Work out the finished part from the listing and answer in its coordinate system (mm). Face numbers are marked on the shaded views. A direction names the side the tool comes from. Coordinates: 2 decimals unless noted, no trailing zeros. Order: outer loops, then holes, each group sorted by start corner. A loop starts at its lowest first (then second) coordinate and runs counter-clockwise, first axis right, second up. Notation, with made-up numbers: M 83,73 L 132,73 A21 ccw 132,84 Z; hole C -5,34.25 d9. An arc over 180 degrees is marked long. Write item = value, one per line. Start each with the question number.
Q1. Determine the mould class of the marked faces 6, 7 and 8 for opening direction X: released by +X, released by -X, zero draft, split by the parting line, or undercut.
Q2. A tool of negligible diameter and unlimited length cuts with its end or side. For the marked faces 1, 2, 3, 4 and 5, from which of +Z, -Z, +X, -X, +Y, -Y can it reach the whole face along a straight path? Write none if from no direction.
Q3. Find section C-C on y = 51. Give the vertices of the cut face in (x, z).
Q4. Find section D-D on y = 101. Give the vertices of the cut face in (x, z), and give its area (3 significant figures).
Q5. Each of these flat-tipped pins is pushed along its axis until it touches: P1, Ø10, axis at y = 42, z = -19, coming from the -X side; P2, Ø3, axis at y = 87, z = -14.5, coming from the +X side; P3, Ø14.5, axis at y = 11.5, z = -42.5, coming from the +X side. Where does it stop, or does it pass through?
Q6. Find section B-B on x = -40. Give the vertices of the cut face in (y, z).
Q7. Straight lines are drawn through the part: line 1 along X through (y, z) = (6.5, -72); line 2 along Z through (x, y) = (57, 103); line 3 along Y through (x, z) = (84, -51). For each, find the intervals that lie inside material, in ascending order.
Q8. Find section A-A on z = -46. Give the vertices of the cut face in (x, y).
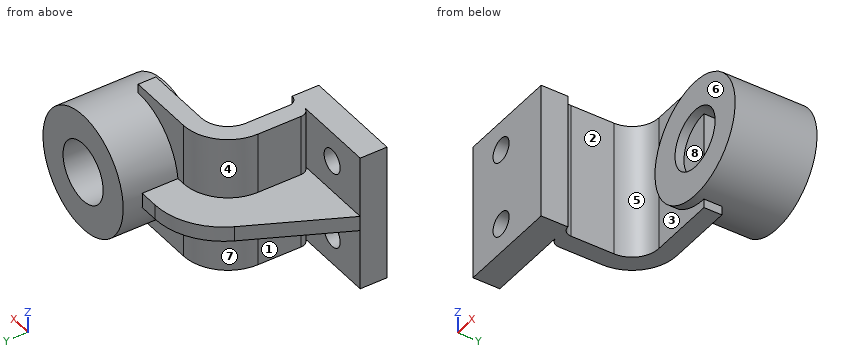
```python
from build123d import *

# Parameters (mm, degrees)
BOSS_EXTRUDE1_DEPTH = 92
BOSS_EXTRUDE2_START = -18
SKETCH2_R           = 40
SKETCH2_R_2         = 20
BOSS_EXTRUDE2_DEPTH = 55
SKETCH3_R           = 8
CUT_EXTRUDE1_DEPTH  = 18
BOSS_EXTRUDE3_START = -46
BOSS_EXTRUDE3_DEPTH = 5
FILLET1_R           = 46


with BuildPart() as part:
    # Sketch1 → Boss-Extrude1 (new body)
    with BuildSketch(Plane.XY):
        with BuildLine():
            Line((-6, 53), (-6, 24))
            ThreePointArc((-6, 24), (-4.242640687, 19.757359313), (0, 18))
            Line((0, 18), (0, 0))
            Line((0, 0), (-68, 0))
            Line((-68, 0), (-68, 18))
            Line((-68, 18), (-12, 18))
            ThreePointArc((-12, 18), (-16.242640687, 19.757359313), (-18, 24))
            Line((-18, 24), (-18, 53))
            ThreePointArc((-18, 53), (-9.213203436, 74.213203436), (12, 83))
            Line((12, 83), (57, 83))
            Line((57, 83), (57, 71))
            Line((57, 71), (12, 71))
            ThreePointArc((12, 71), (-0.727922061, 65.727922061), (-6, 53))
        make_face()
    extrude(amount=-BOSS_EXTRUDE1_DEPTH)

    # Sketch2 → Boss-Extrude2 (add)
    with BuildSketch(Plane(origin=(0, 83, 0), x_dir=(1, 0, 0), z_dir=(0, 1, 0)).offset(BOSS_EXTRUDE2_START)):
        with Locations(Location((57, 46, 0), (0, 0, 90))):
            Circle(SKETCH2_R)
        with Locations(Location((57, 46, 0), (0, 0, 90))):
            Circle(SKETCH2_R_2, mode=Mode.SUBTRACT)
    extrude(amount=BOSS_EXTRUDE2_DEPTH)

    # Sketch3 → Cut-Extrude1 (cut)
    with BuildSketch(Plane(origin=(0, 18, 0), x_dir=(1, 0, 0), z_dir=(0, 1, 0))):
        with Locations(Location((-40, 20, 0), (0, 0, 270))):
            Circle(SKETCH3_R)
        with Locations(Location((-40, 72, 0), (0, 0, 270))):
            Circle(SKETCH3_R)
    extrude(amount=-CUT_EXTRUDE1_DEPTH, mode=Mode.SUBTRACT)

    # Sketch4 → Boss-Extrude3 (add, symmetric)
    with BuildSketch(Plane.XY.offset(BOSS_EXTRUDE3_START)):
        with BuildLine():
            ThreePointArc((-18, 53), (-9.213203436, 74.213203436), (12, 83))
            Line((12, 83), (17, 83))
            Line((17, 83), (18, 83))
            Line((18, 83), (18, 107))
            Line((18, 107), (-24, 107))
            Line((-24, 107), (-68, 18))
            Line((-68, 18), (-12, 18))
            ThreePointArc((-12, 18), (-16.242640687, 19.757359313), (-18, 24))
            Line((-18, 24), (-18, 53))
        make_face()
    extrude(amount=BOSS_EXTRUDE3_DEPTH, both=True)

    # Fillet1
    fillet1_edges = [part.edges().sort_by_distance(p)[0] for p in [
        (-24, 107, -46),
    ]]
    fillet(fillet1_edges, radius=FILLET1_R)


solid = part.part
```
Findings below:
q1.face_6 = zero draft
q1.face_7 = released by -X
q1.face_8 = undercut
q2.face_1 = -Z, -X, +Y
q2.face_2 = +Z, -Z, +X
q2.face_3 = -Y
q2.face_4 = +Z, -X, +Y
q2.face_5 = +Z, -Z
q3.outline = M -51.69,-51 L -18,-51 L -18,-92 L -6,-92 L -6,0 L -18,0 L -18,-41 L -51.69,-41 Z
q4.outline = M -18.14,-51 L 17.31,-51 A40 ccw long 17.31,-41 L -18.14,-41 Z; hole C 57,-46 d40
q4.area = 4,120 mm^2
q5.P1 = -18
q5.P2 = 83.46
q5.P3 = 0
q6.outline = M 0,-92 L 18,-92 L 18,-80 L 0,-80 Z; M 0,-64 L 18,-64 L 18,-51 L 74.64,-51 L 74.64,-41 L 18,-41 L 18,-28 L 0,-28 Z; M 0,-12 L 18,-12 L 18,0 L 0,0 Z
q7.line_1 = -68 to -48, -32 to 0
q7.line_2 = -86 to -66, -26 to -6
q7.line_3 = 65 to 120
q8.outline = M -68,0 L 0,0 L 0,18 A6 cw -6,24 L -6,53 A18 cw 12,71 L 17,71 L 17,65 L 37,65 L 37,71 L 57,71 L 57,83 L 37,83 L 37,120 L 17,120 L 17,107 L 4.57,107 A46 ccw -36.66,81.39 L -68,18 Z; M 77,65 L 97,65 L 97,120 L 77,120 Z
